Part print with two shaded views. Sizes in mm from the minimum x, y, z corner. A direction names the side the tool comes from. Round coordinates to 2 decimals unless told otherwise and drop trailing zeros. Write each loop counter-clockwise with the first axis right and the second up, starting at its lowest first coordinate (ties: lowest second). Pieces come first, ordered by that corner, then holes. Notation, with made-up numbers: M -1.75,52.5 L 53.25,52.5 A34 ccw 53.25,83.5 Z; hole C 10.25,35.25 d11. An arc over 180 degrees is marked long. Use one line per item in the form item = value. Start each with the question number.
Item 1: Flat gauge pins, fed straight in: pin 1 Ø3 at (x, z) = (11, 37.5) entering from +Y; pin 2 Ø5 at (y, z) = (17, 15) entering from -X; pin 3 Ø16 at (x, y) = (58, 35.5) entering from -Z. Where does each tip first touch, or does it go through?
Item 2: Cut at D-D, the plane y = 17. Give the cut face in (x, z), then the cut area to 3 significant figures.
Item 3: Mould opens along X. For the marked faces 1, 2 and 3 say: +X half, -X half, draft (parallel to the pull), parting line (faces both ways), or undercut.
Item 4: Which spindle directions (+Z, -Z, +X, -X, +Y, -Y) get a long thin tool onto all of the face, cutting with end or side? Do the marked faces 4, 5 and 6. Say none if no direction does.
Item 5: Cut at A-A, the plane z = 20. Give the cut face in (x, y).
Item 6: Probe L1, parallel to Y at x = 13.5, z = 45.5; L2, parallel to X at y = 11, z = 17; L3, parallel to Z at x = 41, y = 23. List the from-to ranges inside material, lowest first.
Item 7: Cut at B-B, the plane y = 44. Give the cut face in (x, z), then the cut area to 3 significant figures.
Item 8: Cut at C-C, the plane x = 37.5. Give the cut face in (y, z), then the cut area to 3 significant figures.
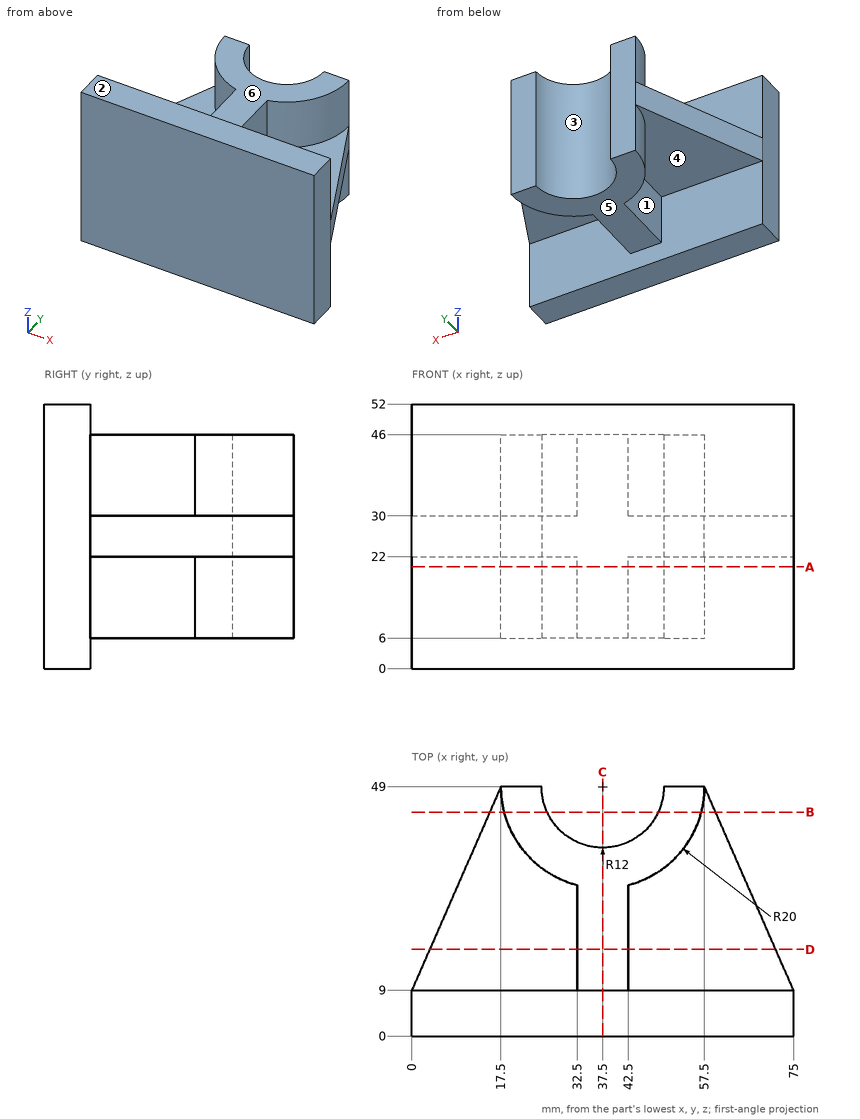
Model answer:
q1.pin_1 = 9
q1.pin_2 = 32.5
q1.pin_3 = 6
q2.outline = M 3.5,22 L 32.5,22 L 32.5,6 L 42.5,6 L 42.5,22 L 71.5,22 L 71.5,30 L 42.5,30 L 42.5,46 L 32.5,46 L 32.5,30 L 3.5,30 Z
q2.area = 864 mm²
q3.face_1 = -X half
q3.face_2 = draft
q3.face_3 = undercut
q4.face_4 = -Z, -X
q4.face_5 = -Z, +X, -X, +Y
q4.face_6 = +Z, +X, -X, +Y
q5.outline = M 0,0 L 75,0 L 75,9 L 42.5,9 L 42.5,29.64 A20 ccw 57.5,49 L 49.5,49 A12 cw 25.5,49 L 17.5,49 A20 ccw 32.5,29.64 L 32.5,9 L 0,9 Z
q6.L1 = 0 to 9
q6.L2 = 32.5 to 42.5
q6.L3 = 6 to 46
q7.outline = M 15.31,22 L 18.14,22 L 18.14,6 L 26.59,6 L 26.59,46 L 18.14,46 L 18.14,30 L 15.31,30 Z; M 48.41,6 L 56.86,6 L 56.86,22 L 59.69,22 L 59.69,30 L 56.86,30 L 56.86,46 L 48.41,46 Z
q7.area = 722 mm²
q8.outline = M 0,0 L 9,0 L 9,6 L 37,6 L 37,46 L 9,46 L 9,52 L 0,52 Z
q8.area = 1,590 mm²
